Could you check a few things on this model? Use its own coordinates, in mm. A direction names the side the tool comes from. Coordinates: 2 decimals unless noted, no trailing zeros. Write each loop counter-clockwise with the first axis right and the second up, starting at its lowest first coordinate (ties: lowest second). Pieces come first, ordered by that corner, then holes.
Item 1: If I drill on probe 1 along Y at (x, z) = (160, -20); probe 2 along Z at (x, y) = (-36.5, -6); probe 3 along Z at (x, y) = (-60.5, -6.25), over which ranges is the centre line in solid material (lowest first)?
Item 2: Which directions (+Z, -Z, +X, -X, +Y, -Y) give clear straight access to the entire face, cutting with the end or side of a thin tool? Please do faces 1 (the flat face through (-3, 9, 0)), 2 (the flat face through (-3, -9, 0)), 3 (the flat face through (-60, 0, 29)).
Item 3: I want a section at C-C on x = -150. Please give me the cut outline in (y, z).
Item 4: I want a section at B-B on z = -154.5. Please give me the cut outline in (x, y), then the cut area to 3 significant figures.
Item 5: Thinking about a two-plate mould opening in Z: for faces 4 (the cylindrical face through (-152.23, -0.04, -354.89)), 5 (the flat face through (1, -15, 11)), 6 (the flat face through (30, 0, 20)), which applies, +Z half, -Z half, draft (parallel to the pull), parting line (faces both ways), or undercut?
Item 6: For P1, Ø3, axis at x = 1, y = -6.5, coming from the +Z side; P2, Ø3, axis at x = 26, y = -10, coming from the -Z side; P3, Ø5, axis at x = -35, z = -304.5, coming from the +Y side; P4, Ø14, axis at x = -47, y = 8.5, coming from the -Z side, each with a flat end and sliding along its axis, tell me the tip position at first contact or that it passes through.
Item 7: I want a section at D-D on z = 14.5. Please give me the cut outline in (x, y).
Autodesk Inventor part; units mm, degrees
ref_plane "YZ Plane" through (0, 0, 0) normal (1, 0, 0) x (0, 1, 0)
ref_plane "XZ Plane" through (0, 0, 0) normal (0, 1, 0) x (-1, 0, 0)
ref_plane "XY Plane" through (0, 0, 0) normal (0, 0, 1) x (1, 0, 0)
sketch "panel_sketch" plane through (0, 0, 0) normal (0, 1, 0) x (-1, 0, 0)
  line L0 (195, 0) -> (195, -250)
  line L1 (195, 0) -> (0, 0)
  line L2 (0, 0) -> (0, -400)
  line L3 (0, -400) -> (45, -400)
  arc A0 (45, -400) -> (195, -250) centre (45, -250) ccw
  line L4 (-195, 0) -> (-195, -250)
  line L5 (-195, 0) -> (0, 0)
  line L6 (0, -400) -> (-45, -400)
  arc A1 (-195, -250) -> (-45, -400) centre (-45, -250) ccw
  dimension "d1" = 400
  dimension "d2" = 390
  dimension "d3" = 250
  dimension "d4" = 45
extrude "panel_extrude" add sketch "panel_sketch" along normal mid plane 5
sketch "hinge_sketch" plane through (0, 0, 0) normal (0, 1, 0) x (-1, 0, 0)
  line L0 (195, -250) -> (195, 0)
  line L1 (195, 0) -> (195, 5)
  line L2 (195, 5) -> (30, 5)
  line L3 (30, 5) -> (30, 45)
  line L4 (0, 0) -> (0, 150)
  line L5 (195, 0) -> (0, 0)
  line L6 (195, 0) -> (-195, 0)
  line L7 (30, 45) -> (0, 45)
  line L8 (-195, 0) -> (-195, 5)
  line L9 (-195, 5) -> (-30, 5)
  line L10 (-30, 5) -> (-30, 45)
  line L11 (-195, 0) -> (0, 0)
  line L12 (-30, 45) -> (0, 45)
  dimension "d8" = 5
  dimension "d9" = 60
  dimension "d10" = 40
  dimension "d19" = 150
extrude "hinge_extrude" add sketch "hinge_sketch" along normal mid plane 30
fillet "hinge_bottom_fillet" radius 15 2 edges at (0, 15, 45) (0, -15, 45)
sketch "hinge_link_sketch" plane through (-30, -15, 5) normal (-1, 0, 0) x (0, 0, 1)
  line L0 (0, 30) -> (25, 30)
  arc A0 (25, 0) -> (25, 30) centre (25, 15) ccw
  line L1 (25, 0) -> (0, 0)
  circle A1 centre (24, 15) radius 7.5
  point P0 (-5, 15)
  point P1 (40, 15)
  dimension "d14" = 15
  dimension "d15" = 16
  dimension "d16" = 15
extrude "hinge_link_extrude" add sketch "hinge_link_sketch" along normal blind 30
mirror "hinge_link_extrude_mirror" about plane through (0, 0, 0) normal (1, 0, 0)
equation "\"d1\" = panel_height"
equation "\"d2\" = panel_width"
equation "\"d3\" = vertical_height"
equation "\"d4\" = 0.5 * panel_width + vertical_height - panel_height"
equation "\"d9\" = hinge_width"
equation "\"d10\" = hinge_height"
equation "\"d11\" = 0.5 * hinge_width"
equation "\"d17\" = 0.5 * hinge_width"
equation "\"panel_height\" = 400"
equation "\"panel_width\" = 390"
equation "\"vertical_height\" = 250"
equation "\"hinge_width\" = 60"
equation "\"hinge_height\" = 40"
properties part number "aperature_panel" material "Stainless Steel AISI 440C, Welded"
Response values:
1. probe 1: y = -2.5 to 2.5
1. probe 2: z = 0 to 5, 24.5 to 33.5
1. probe 3: z = 0 to 5
2. face 1: -Z, +X, -X, +Y
2. face 2: -Z, +X, -X, -Y
2. face 3: +Z, -X, +Y, -Y
3. outline: (-15, 0) - (-2.5, 0) - (-2.5, -357.12) - (2.5, -357.12) - (2.5, 0) - (15, 0) - (15, 5) - (-15, 5) - close
4. outline: (-195, -2.5) - (195, -2.5) - (195, 2.5) - (-195, 2.5) - close
4. area: 1,950 mm2
5. face 4: -Z half
5. face 5: draft
5. face 6: undercut
6. P1: stops at z = 44.14
6. P2: stops at z = 0
6. P3: stops at y = 2.5
6. P4: stops at z = -400
7. outline: (-30, -15) - (30, -15) - (30, 15) - (-30, 15) - close
